Part print with two shaded views. Sizes in mm from the minimum x, y, z corner. Round coordinates to 2 decimals unless told otherwise and drop trailing zeros. Loops run counter-clockwise (first coordinate to the right, second up) from the corner with the lowest first, then second, coordinate; pieces in that order, holes last. Notation, with made-up numbers: (57.5, -9) -> (113.5, -9) arc R22 cw to (113.5, 24) -> close; hole circle Ø5 at (5, -8.5). An arc over 180 degrees is marked (long way). Put each result on its own line as item: value. Start each with the question number.
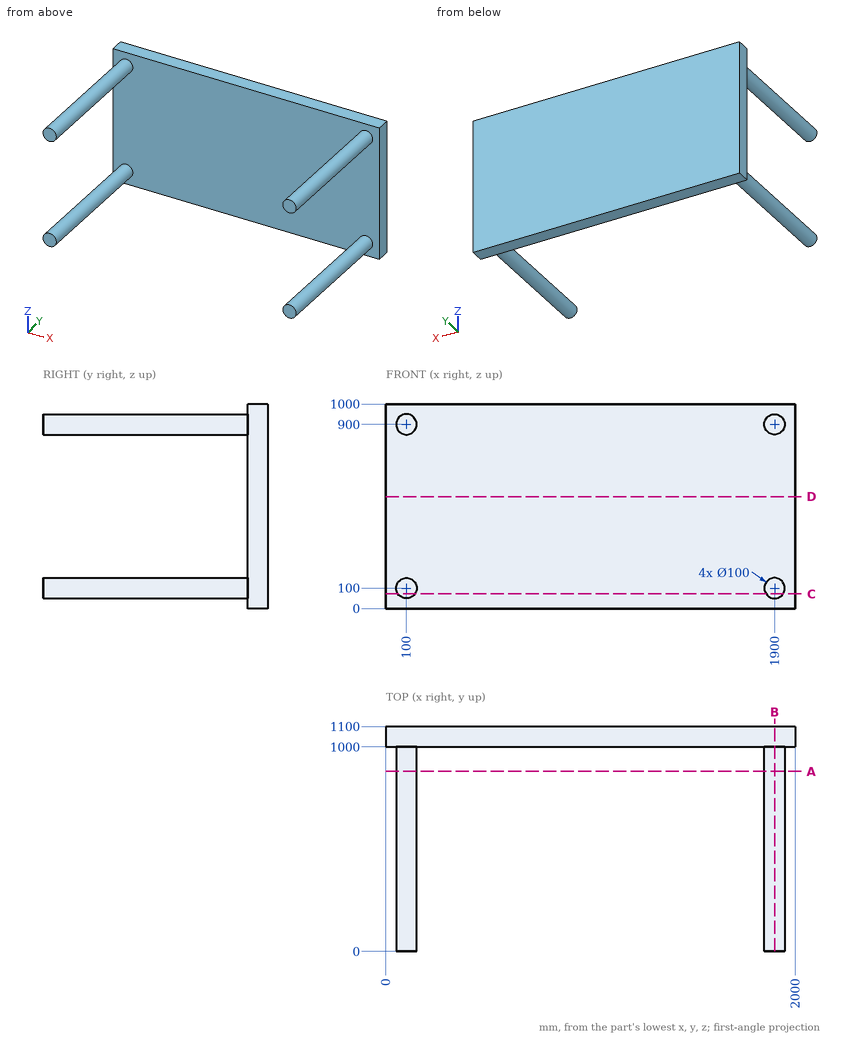
Item 1: Cut at A-A on y = 881. Write the cut outline in (x, z).
Item 2: Cut at C-C on z = 71. Write the cut outline in (x, y), then the cut area to 3 significant figures.
Item 3: Cut at B-B on x = 1900. Write the cut outline in (y, z).
Item 4: Wall check: line 1 (X direction, y = 594, z = 895); line 2 (Y direction, x = 1230, z = 875); line 3 (X direction, y = 651.5, z = 883.5). Give the ranges that are in metal, low to high. Write a range as from..to.
Item 5: Cut at D-D on z = 547. Write the cut outline in (x, y).
Ans:
1. outline: circle Ø100 at (100, 100); circle Ø100 at (100, 900); circle Ø100 at (1900, 100); circle Ø100 at (1900, 900)
2. outline: (0, 1000) -> (59.27, 1000) -> (59.27, 0) -> (140.73, 0) -> (140.73, 1000) -> (1859.27, 1000) -> (1859.27, 0) -> (1940.73, 0) -> (1940.73, 1000) -> (2000, 1000) -> (2000, 1100) -> (0, 1100) -> close
2. area: 363,000 mm2
3. outline: (0, 50) -> (1000, 50) -> (1000, 0) -> (1100, 0) -> (1100, 1000) -> (1000, 1000) -> (1000, 950) -> (0, 950) -> (0, 850) -> (1000, 850) -> (1000, 150) -> (0, 150) -> close
4. line 1: x = 50.25..149.75, 1850.25..1949.75
4. line 2: y = 1000..1100
4. line 3: x = 52.8..147.2, 1852.8..1947.2
5. outline: (0, 1000) -> (2000, 1000) -> (2000, 1100) -> (0, 1100) -> close
